Design review of the part built by this model. Coordinates are the model's own, in mm. Face numbers are marked on the shaded views. A direction names the side the tool comes from. Round coordinates to 2 decimals unless told otherwise and drop trailing zeros. Loops run counter-clockwise (first coordinate to the right, second up) from the corner with the lowest first, then second, coordinate; pieces in that order, holes last. Notation, with made-up numbers: (62, -21) - (87, -21) arc R16 cw to (87, -6) - close; hole circle Ø10 at (-13.75, 53.25). An arc over 180 degrees is marked (long way). Return JSON: item names as keys, results as strings. Group by question number.
(1) We need section B-B, the plane y = 15.5. Write out the cut boundary in (x, z).
(2) We need section A-A, the plane x = 25.4. Write out the cut boundary in (y, z) (3 decimals), and give its area (3 significant figures).
(3) We need section C-C, the plane x = 6. Write out the cut boundary in (y, z) (3 decimals), and give its area (3 significant figures).
(4) Wall thickness on L1, parallel to Y at x = 25.4, z = -45.5 (3 decimals); L2, parallel to X at y = 3.75, z = -7.5; L3, parallel to Z at x = 23.5, y = 4.75: over which ranges is each line inside the solid? List them lowest first. Write a range as [from, to].
(5) For the marked faces 5, 6 and 7, list the 3-axis set-ups (+Z, -Z, +X, -X, +Y, -Y) from which the entire face can be reached by the end or side of a thin tool; tool diameter is ignored.
(6) Clearance check with flat-ended pins moving along their axes: pin 1 (5 mm diameter, centred on y = 16, z = -37, fed in from -X); pin 2 (3 mm diameter, centred on x = 45, y = 7, fed in from +Z); pin 3 (3.5 mm diameter, centred on y = 9, z = -7.5, fed in from +X); pin 4 (3.5 mm diameter, centred on x = 6.5, y = 1.5, fed in from +Z). State where each tip first meets the part, or that it passes through.
(7) We need section D-D, the plane y = 5.75. Write out the cut boundary in (x, z).
(8) The part is to be moulded in two halves that separate along Z. For the marked faces 1, 2, 3 and 4, say which applies: pulls with the +Z half, pulls with the -Z half, needs draft (parallel to the pull), parting line crosses it, or undercut.
Autodesk Inventor part; units mm, degrees
ref_plane "YZ Plane" through (0, 0, 0) normal (1, 0, 0) x (0, 1, 0)
ref_plane "XZ Plane" through (0, 0, 0) normal (0, 1, 0) x (-1, 0, 0)
ref_plane "XY Plane" through (0, 0, 0) normal (0, 0, 1) x (1, 0, 0)
sketch "Sketch1" plane through (0, 0, 0) normal (0, 0, 1) x (1, 0, 0)
  line L0 (0, 0) -> (50.8, 0)
  line L1 (50.8, 0) -> (50.8, 18.669)
  line L2 (50.8, 18.669) -> (0, 18.669)
  line L3 (0, 18.669) -> (0, 0)
  dimension "d0" = 50.8
  dimension "d1" = 18.669
extrude "Extrusion1" add sketch "Sketch1" against normal blind 50.8
sketch "Sketch2" plane through (0, 0, 0) normal (0, 0, 1) x (1, 0, 0)
  line L0 (50.8, 0) -> (0, 0)
  line L1 (25.4, 0) -> (25.4, 3.175)
  line L2 (25.4, 3.175) -> (26.9875, 3.175)
  line L3 (25.4, 3.175) -> (23.8125, 3.175)
  line L4 (23.8125, 3.175) -> (23.8125, 18.669)
  line L5 (0, 18.669) -> (50.8, 18.669)
  line L6 (26.9875, 3.175) -> (26.9875, 18.669)
  line L7 (23.8125, 18.669) -> (12.1285, 18.669)
  line L8 (12.1285, 18.669) -> (12.1285, 0)
  line L9 (12.1285, 0) -> (25.4, 0)
  line L10 (26.9875, 18.669) -> (38.6715, 18.669)
  line L11 (38.6715, 18.669) -> (38.6715, 0)
  line L12 (38.6715, 0) -> (25.4, 0)
  line L13 (0, 0) -> (0, 18.669)
  line L14 (0, 18.669) -> (0, 0)
  line L15 (50.8, 18.669) -> (50.8, 0)
  line L16 (50.8, 18.669) -> (50.8, 0)
  dimension "d4" = 3.175
  dimension "d5" = 1.5875
  dimension "d6" = 1.5875
  dimension "d15" = 11.684
  dimension "d16" = 11.684
sketch "Sketch3" plane through (0, 0, 0) normal (-1, 0, 0) x (0, 0, 1)
  line L0 (0, 0) -> (-50.8, 0)
  line L1 (0, 0) -> (0, 3.175)
  line L2 (0, 0) -> (0, 18.669)
  line L3 (0, 3.175) -> (-11.684, 3.175)
  line L4 (-50.8, 18.669) -> (-50.8, 0)
  line L5 (-50.8, 0) -> (-50.8, 3.175)
  line L6 (-50.8, 3.175) -> (-39.116, 3.175)
  line L7 (0, 18.669) -> (-50.8, 18.669)
  line L8 (-39.116, 3.175) -> (-11.684, 3.175)
  line L9 (-11.684, 3.175) -> (-11.684, 18.669)
  line L10 (-11.684, 18.669) -> (-39.116, 18.669)
  line L11 (-39.116, 18.669) -> (-39.116, 3.175)
  dimension "d7" = 3.175
  dimension "d8" = 11.684
  dimension "d9" = 3.175
  dimension "d10" = 11.684
extrude "Extrusion2" cut sketch "Sketch3" against normal blind 50.8 contours L8 L11 L7 L9
extrude "Extrusion3" cut sketch "Sketch2" against normal up to surface (11.684 mm away) contours L0 L11 L5 L15 | L0 L13 L5 L8
extrude "Extrusion4" cut sketch "Sketch2" against normal up to surface (11.684 mm away) contours L3 L4 L5 L6 L2
sketch "Sketch5" plane through (38.6715, 0, 0) normal (1, 0, 0) x (0, 0, -1)
  line L0 (0, 18.669) -> (11.684, 18.669)
  circle A0 centre (5.842, 9.3345) radius 2
  point P0 (0, 0)
  dimension "d21" = 4
extrude "Extrusion5" cut sketch "Sketch5" against normal up to surface (11.684 mm away)
sketch "Sketch6" plane through (0, 0, -50.8) normal (0, 0, -1) x (-1, 0, 0)
  line L0 (-50.8, 18.669) -> (-50.8, 0)
  line L1 (0, 18.669) -> (-50.8, 18.669)
  line L2 (-12.1285, 0) -> (-38.6715, 0)
  circle A0 centre (-25.4, 6.985) radius 2
  circle A1 centre (-25.4, 14.732) radius 2
  point P0 (0, 0)
  dimension "d25" = 4
  dimension "d27" = 4
extrude "Extrusion6" cut sketch "Sketch6" against normal up to surface (11.684 mm away)
properties part number "Slit holder"
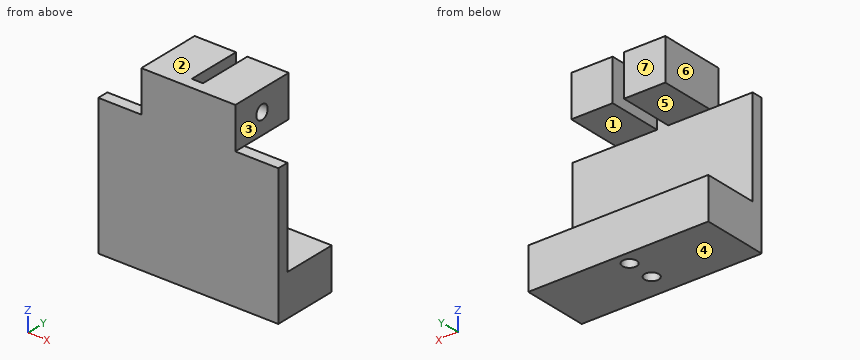
Solutions:
{
 "1": {"outline": "(0, -50.8) - (23.55, -50.8) - (23.55, -39.12) - (0, -39.12) - close; (12.13, -11.68) - (23.81, -11.68) - (23.81, 0) - (12.13, 0) - close; (26.99, -11.68) - (38.67, -11.68) - (38.67, 0) - (26.99, 0) - close; (27.25, -50.8) - (50.8, -50.8) - (50.8, -39.12) - (27.25, -39.12) - close"},
 "2": {"outline": "(0, -50.8) - (4.985, -50.8) - (4.985, -39.116) - (3.175, -39.116) - (3.175, 0) - (0, 0) - close; (8.985, -50.8) - (12.732, -50.8) - (12.732, -39.116) - (8.985, -39.116) - close; (16.732, -50.8) - (18.669, -50.8) - (18.669, -39.116) - (16.732, -39.116) - close", "area": "249 mm^2"},
 "3": {"outline": "(0, -50.8) - (18.669, -50.8) - (18.669, -39.116) - (3.175, -39.116) - (3.175, -11.684) - (0, -11.684) - close", "area": "305 mm^2"},
 "4": {"L1": "[0, 4.985], [8.985, 12.732], [16.732, 18.669]", "L2": "[12.13, 23.81], [26.99, 38.67]", "L3": "[-50.8, -39.12], [-11.68, 0]"},
 "5": {"face 5": "+X, -X, +Y", "face 6": "+Z, -X, +Y, -Y", "face 7": "+Z, -Z, +X, -X, +Y"},
 "6": {"pin 1": "x = 0", "pin 2": "z = -39.12", "pin 3": "x = 38.67", "pin 4": "z = -11.68"},
 "7": {"outline": "(0, -50.8) - (23.83, -50.8) - (23.83, -39.12) - (0, -39.12) - close; (12.13, -11.68) - (23.81, -11.68) - (23.81, 0) - (12.13, 0) - close; (26.97, -50.8) - (50.8, -50.8) - (50.8, -39.12) - (26.97, -39.12) - close; (26.99, -11.68) - (38.67, -11.68) - (38.67, 0) - (26.99, 0) - close"},
 "8": {"face 1": "undercut", "face 2": "pulls with the +Z half", "face 3": "needs draft", "face 4": "pulls with the -Z half"}
}
